Could you check a few things on this model? Use its own coordinates, in mm. A direction names the side the tool comes from. Coordinates: 2 decimals unless noted, no trailing zeros. Write each loop counter-clockwise with the first axis right and the second up, starting at its lowest first coordinate (ties: lowest second). Pieces come first, ordered by that corner, then holes. Notation, with made-up numbers: (-10.75, -23.75) - (23.25, -23.75) arc R31 cw to (23.25, 9.25) - close; hole circle Ø9 at (32.5, -36). An arc over 180 degrees is marked (long way). Answer as a JSON object with one key per item and string values. Group by question number.
1) Please list where these lines run through material, in increasing order: line 1 along X through (y, z) = (-33, -6); line 2 along Y through (x, z) = (5, 12); line 3 along Z through (x, y) = (-6.35, -35).
2) If we section it at D-D (x = 9): Write out the boundary of the cut face in (y, z), plus the area to 3 significant figures.
3) Will these pins go through, and if not, where does the flat tip stop? pin 1 Ø7.5 at (x, z) = (-6.35, -6.35) entering from -Y; pin 2 Ø1.9 at (y, z) = (-43, 15.5) entering from +X; pin 3 Ø7 at (y, z) = (-4.5, 15.5) entering from -X; pin 4 Ø8 at (x, z) = (-15.5, 7) entering from +Y.
4) If we section it at A-A (y = -28): Write out the boundary of the cut face in (x, z).
5) If we section it at C-C (x = -6.35): Write out the boundary of the cut face in (y, z).
6) On a 3-axis mill with a long thin cutter (end or side, diameter ignored), from which of +Z, -Z, +X, -X, +Y, -Y can I reach the whole of each face in a straight line? I mean faces 1 (the flat face through (7.202, -6, 16)), 2 (the flat face through (-6, -12.7, 11)), 3 (the flat face through (19.05, -26, 3)). Say none if no direction works.
7) If we section it at B-B (z = 11): Write out the boundary of the cut face in (x, y).
8) We'd pull the mould along X, two halves only. Please class faces 4 (the flat face through (32, -26, -6.35)), 5 (the flat face through (-44.45, -25, -13)), 6 (the flat face through (-6, -45, 12.7)): released by +X, released by -X, zero draft, split by the parting line, or undercut.
```python
from build123d import *

# Parameters (mm, degrees)
F0_W      = 88.9
F0_H      = 38.1
F1_DEPTH  = 50.8
F2_W      = 12.7
F2_H      = 25.4
F3_DEPTH  = 50.801
F4_W      = 25.4
F4_H      = 25.4
F5_DEPTH  = 50.801
F6_W      = 25.4
F6_H      = 6.35
F7_DEPTH  = 50.801
F8_R      = 6.35
F9_DEPTH  = 50.801
F10_W     = 25.4
F10_H     = 12.7
F11_DEPTH = 63.501


with BuildPart() as f1:
    # F0 (on Front) → F1 (new body)
    with BuildSketch(Plane.XZ):
        Rectangle(F0_W, F0_H)
    extrude(amount=F1_DEPTH)

    # F2 (on face) → F3 (cut, through all)
    with BuildSketch(Plane.XZ.offset(50.8)):
        with Locations((-38.1, 6.35)):
            Rectangle(F2_W, F2_H)
    extrude(amount=-F3_DEPTH, mode=Mode.SUBTRACT)

    # F4 (on face) → F5 (cut, through all)
    with BuildSketch(Plane.XZ.offset(50.8)):
        with Locations((31.75, 6.35)):
            Rectangle(F4_W, F4_H)
    extrude(amount=-F5_DEPTH, mode=Mode.SUBTRACT)

    # F6 (on face) → F7 (cut, through all)
    with BuildSketch(Plane.XZ.offset(50.8)):
        with Locations((-5.497764, 15.875)):
            Rectangle(F6_W, F6_H)
    extrude(amount=-F7_DEPTH, mode=Mode.SUBTRACT)

    # F8 (on face) → F9 (cut, through all)
    with BuildSketch(Plane.XZ.offset(50.8)):
        with Locations((-6.35, -6.35)):
            Circle(F8_R)
    extrude(amount=-F9_DEPTH, mode=Mode.SUBTRACT)

    # F10 (on face) → F11 (cut, through all)
    with BuildSketch(Plane.YZ.offset(19.05)):
        with Locations((-25.4, 12.783553)):
            Rectangle(F10_W, F10_H)
    extrude(amount=-F11_DEPTH, mode=Mode.SUBTRACT)


solid = f1.part
```
Here are the results:
{
 "1": {"line 1": "x = -31.75 to -12.69, -0.01 to 19.05", "line 2": "y = -50.8 to -38.1, -12.7 to 0", "line 3": "z = -19.05 to -12.7, 0 to 6.43"},
 "2": {"outline": "(-50.8, -19.05) - (0, -19.05) - (0, 19.05) - (-12.7, 19.05) - (-12.7, 6.43) - (-38.1, 6.43) - (-38.1, 19.05) - (-50.8, 19.05) - close", "area": "1,620 mm²"},
 "3": {"pin 1": "passes through", "pin 2": "stops at x = 19.05", "pin 3": "stops at x = -31.75", "pin 4": "stops at y = 0"},
 "4": {"outline": "(-44.45, -19.05) - (44.45, -19.05) - (44.45, -6.35) - (19.05, -6.35) - (19.05, 6.43) - (-31.75, 6.43) - (-31.75, -6.35) - (-44.45, -6.35) - close; hole circle Ø12.7 at (-6.35, -6.35)"},
 "5": {"outline": "(-50.8, -19.05) - (0, -19.05) - (0, -12.7) - (-50.8, -12.7) - close; (-50.8, 0) - (0, 0) - (0, 12.7) - (-12.7, 12.7) - (-12.7, 6.43) - (-38.1, 6.43) - (-38.1, 12.7) - (-50.8, 12.7) - close"},
 "6": {"face 1": "+Z, +Y, -Y", "face 2": "+Z, +X, -X", "face 3": "+Z, +X, +Y, -Y"},
 "7": {"outline": "(-31.75, -50.8) - (19.05, -50.8) - (19.05, -38.1) - (-31.75, -38.1) - close; (-31.75, -12.7) - (19.05, -12.7) - (19.05, 0) - (-31.75, 0) - close"},
 "8": {"face 4": "zero draft", "face 5": "released by -X", "face 6": "undercut"}
}
